Can you work these out from the model? Positions are in its coordinate system, mm. Give positions to 0.01 mm unless a question says otherwise; leave off trailing zeros. Loops run counter-clockwise (first coordinate to the right, second up) from the corner with the lowest first, then second, coordinate; pieces in that order, holes last. Notation, with made-up numbers: (-28.75, -7.75) -> (17.25, -7.75) arc R12 cw to (17.25, 15.25) -> close; hole circle Ø6 at (-30, -20.5). An arc over 180 degrees is marked (long way). Return JSON: item names as keys, results as strings. Group by question number.
Q1. I need wall thicknesses on line 1 along X through (y, z) = (1.15, 0); line 2 along X through (y, z) = (2.55, -1); line 3 along X through (y, z) = (1, 20). Which ranges of each line are inside material? Lowest first, please. Write a range as [from, to].
Q2. Will these pins go through, and if not, where does the flat tip stop? pin 1 (1 mm diameter, centred on x = -47, z = -6.5, fed in from -Y); pin 2 (1 mm diameter, centred on x = 1, y = 0.5, fed in from -Z); pin 3 (1.5 mm diameter, centred on x = 97, y = 1, fed in from +Z); pin 4 (1 mm diameter, centred on x = 50.5, y = 2, fed in from +Z).
Q3. Suppose I cut it at B-B, the plane x = 100.5. Please give me the cut outline in (y, z).
Q4. Suppose I cut it at A-A, the plane y = 2.3. Count the separate pieces of the cut face and the enclosed holes in it, and give its area (3 significant figures).
Q5. Suppose I cut it at C-C, the plane z = 41. Please give me the cut outline in (x, y).
```python
from build123d import *

# Parameters (mm, degrees)
SKETCH1_R           = 1.65
BOSS_EXTRUDE1_DEPTH = 3
BOSS_EXTRUDE2_START = -3
BOSS_EXTRUDE2_DEPTH = 3
FILLET1_R           = 10
FILLET2_R           = 3


with BuildPart() as part:
    # Sketch1 → Boss-Extrude1 (new body)
    with BuildSketch(Plane(origin=(0, 0, 0), x_dir=(1, 0, 0), z_dir=(0, 1, 0))):
        with BuildLine():
            Line((62.83311229, -26), (112.579, -26))
            Line((112.579, -26), (112.579, 26))
            Line((112.579, 26), (62.83311229, 26))
            ThreePointArc((62.83311229, 26), (-68, 0), (62.83311229, -26))
        make_face()
        with Locations(Location((86.579, 0, 0), (0, 0, 270))):
            Circle(SKETCH1_R, mode=Mode.SUBTRACT)
        with Locations(Location((94.579, 0, 0), (0, 0, 270))):
            Circle(SKETCH1_R, mode=Mode.SUBTRACT)
        with Locations(Location((106.579, 0, 0), (0, 0, 270))):
            Circle(SKETCH1_R, mode=Mode.SUBTRACT)
        with Locations(Location((86.579, -8, 0), (0, 0, 270))):
            Circle(SKETCH1_R, mode=Mode.SUBTRACT)
        with Locations(Location((86.579, -20, 0), (0, 0, 270))):
            Circle(SKETCH1_R, mode=Mode.SUBTRACT)
        with Locations(Location((78.579, 0, 0), (0, 0, 270))):
            Circle(SKETCH1_R, mode=Mode.SUBTRACT)
        with Locations(Location((66.579, 0, 0), (0, 0, 270))):
            Circle(SKETCH1_R, mode=Mode.SUBTRACT)
        with Locations(Location((86.579, 8, 0), (0, 0, 270))):
            Circle(SKETCH1_R, mode=Mode.SUBTRACT)
        with Locations(Location((86.579, 20, 0), (0, 0, 270))):
            Circle(SKETCH1_R, mode=Mode.SUBTRACT)
    extrude(amount=BOSS_EXTRUDE1_DEPTH)

    # Sketch2 → Boss-Extrude2 (add)
    with BuildSketch(Plane(origin=(0, 3, 0), x_dir=(1, 0, 0), z_dir=(0, 1, 0)).offset(BOSS_EXTRUDE2_START)):
        with BuildLine():
            ThreePointArc((62.83311229, -26), (57.335321786, -36.560373025), (50.079936102, -46))
            Line((50.079936102, -46), (82.83311229, -26))
            Line((82.83311229, -26), (62.83311229, -26))
        make_face()
        with BuildLine():
            Line((62.83311229, 26), (82.83311229, 26))
            Line((82.83311229, 26), (50.079936102, 46))
            ThreePointArc((50.079936102, 46), (57.335321786, 36.560373025), (62.83311229, 26))
        make_face()
    extrude(amount=BOSS_EXTRUDE2_DEPTH)

    # Fillet1
    fillet1_edges = [part.edges().sort_by_distance(p)[0] for p in [
        (50.079936102, 1.5, 46),
        (82.83311229, 1.5, 26),
        (50.079936102, 1.5, -46),
        (82.83311229, 1.5, -26),
    ]]
    fillet(fillet1_edges, radius=FILLET1_R)

    # Fillet2
    fillet2_edges = [part.edges().sort_by_distance(p)[0] for p in [
        (112.579, 1.5, -26),
        (112.579, 1.5, 26),
    ]]
    fillet(fillet2_edges, radius=FILLET2_R)


solid = part.part
```
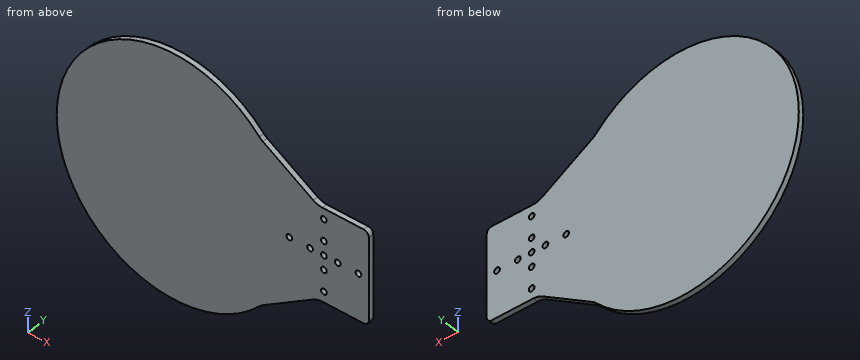
Ans:
{
 "1": {"line 1": "x = [-68, 64.93], [68.23, 76.93], [80.23, 84.93], [88.23, 92.93], [96.23, 104.93], [108.23, 112.58]", "line 2": "x = [-67.99, 65.27], [67.89, 77.27], [79.89, 85.27], [87.89, 93.27], [95.89, 105.27], [107.89, 112.58]", "line 3": "x = [-64.99, 84.93], [88.23, 112.58]"},
 "2": {"pin 1": "stops at y = 0", "pin 2": "stops at z = -68", "pin 3": "stops at z = 26", "pin 4": "stops at z = 46.19"},
 "3": {"outline": "(0, -26) -> (3, -26) -> (3, 26) -> (0, 26) -> close"},
 "4": {"separate pieces": "1", "enclosed holes": "9", "area": "17,200 mm^2"},
 "5": {"outline": "(-54.25, 0) -> (58.27, 0) -> (58.27, 3) -> (-54.25, 3) -> close"}
}
